from build123d import *

# Parameters (mm, degrees)
F0_W      = 24.5
F0_H      = 24.5
F1_DEPTH  = 58
F2_W      = 20.3
F2_H      = 20.3
F3_DEPTH  = 6
F4_W      = 20.5
F4_H      = 20.5
F5_DEPTH  = 30
F7_D      = 5.5
F8_W      = 6.4
F8_H      = 10
F9_DEPTH  = 25
F10_DEPTH = 5
F11_DEPTH = 0.25
F12_DEPTH = 0.25
F13_DEPTH = 1.5
F14_DEPTH = 1
F15_DEPTH = 1
F16_DEPTH = 2


with BuildPart() as f1:
    # F0 (on Top) → F1 (new body)
    with BuildSketch(Plane.XY):
        Rectangle(F0_W, F0_H)
    extrude(amount=F1_DEPTH)

    # F2 (on face) → F3 (cut)
    with BuildSketch(Plane(origin=(0, 0, 0), x_dir=(1, 0, 0), z_dir=(0, 0, -1))):
        Rectangle(F2_W, F2_H)
    extrude(amount=-F3_DEPTH, mode=Mode.SUBTRACT)

    # F4 (on face) → F5 (cut)
    with BuildSketch(Plane.XY.offset(58)):
        with Locations((2, 2)):
            Rectangle(F4_W, F4_H)
    extrude(amount=-F5_DEPTH, mode=Mode.SUBTRACT)

    # F7 (through all)
    with Locations(Plane.YZ.offset(-8.25)):
        with Locations((2, 43)):
            Hole(F7_D / 2)

    # F8 (on face) → F9 (cut)
    with BuildSketch(Plane(origin=(0, -8.25, 0), x_dir=(-1, 0, 0), z_dir=(0, 1, 0))):
        with Locations((-2.0447701301, 43.8107866645)):
            Rectangle(F8_W, F8_H)
    extrude(amount=-F9_DEPTH, mode=Mode.SUBTRACT)

    # F10 (add): a face of the model
    f10_faces = [f1.faces().sort_by_distance(p)[0] for p in [
        (2, 2, 28),
    ]]
    extrude(f10_faces, amount=F10_DEPTH)

    # F11 (cut): a face of the model
    f11_faces = [f1.faces().sort_by_distance(p)[0] for p in [
        (-1.1552298699, -10.25, 43.8107866645),
    ]]
    extrude(f11_faces, amount=-F11_DEPTH, mode=Mode.SUBTRACT)

    # F12 (cut): a face of the model
    f12_faces = [f1.faces().sort_by_distance(p)[0] for p in [
        (5.2447701301, -10.25, 43.8107866645),
    ]]
    extrude(f12_faces, amount=-F12_DEPTH, mode=Mode.SUBTRACT)

    # F13 (cut): a face of the model
    f13_faces = [f1.faces().sort_by_distance(p)[0] for p in [
        (2.0447701301, -10.25, 48.8107866645),
    ]]
    extrude(f13_faces, amount=-F13_DEPTH, mode=Mode.SUBTRACT)

    # F14 (cut): a face of the model
    f14_faces = [f1.faces().sort_by_distance(p)[0] for p in [
        (-12.25, -0.0340074224, 28.7619480432),
    ]]
    extrude(f14_faces, amount=-F14_DEPTH, mode=Mode.SUBTRACT)

    # F15 (cut): a face of the model
    f15_faces = [f1.faces().sort_by_distance(p)[0] for p in [
        (0.4045086201, -12.25, 28.0380957256),
    ]]
    extrude(f15_faces, amount=-F15_DEPTH, mode=Mode.SUBTRACT)

    # F16 (cut): a face of the model
    f16_faces = [f1.faces().sort_by_distance(p)[0] for p in [
        (0, 0, 6),
    ]]
    extrude(f16_faces, amount=-F16_DEPTH, mode=Mode.SUBTRACT)


solid = f1.part
Model file for the job. Use its own axes, mm. A direction names the side the tool comes from. Give positions to 0.01 mm unless a question says otherwise; leave off trailing zeros. Order: outer loops, then holes, each group sorted by start corner. A loop starts at its lowest first (then second) coordinate and runs counter-clockwise, first axis right, second up. Notation, with made-up numbers: (83.5, -29) - (106.5, -29) arc R29 cw to (106.5, -1) - close; hole circle Ø5 at (57.25, 17). An arc over 180 degrees is marked (long way). Write item = value, one per line. Start each with the question number.
1. Cut at B-B, the plane y = 2. List the corners of the cut face in (x, z), and give its area (3 significant figures).
2. Probe line 1 along Z through (x, y) = (-10.2, 2); line 2 along Z through (x, y) = (-9.5, 2); line 3 along Y through (x, z) = (8.5, 4.5). List the from-to ranges inside material, lowest first.
3. Drop flat-ended pins along their axis: P1, Ø10, axis at x = 3.5, y = 2, coming from the -Z side; P2, Ø1, axis at x = -5.5, y = -5, coming from the +Z side; P3, Ø5, axis at x = 9, y = -3.5, coming from the -Z side. Give the stop position or say it passes through.
4. Two-plate mould, pull along X, no slides. Class faces 1 (the flat face through (11, 2, 0)), 2 (the flat face through (10.15, 0, 4)), 3 (the flat face through (-8.25, 0, 46)): pulls with the +X half, pulls with the -X half, needs draft (parallel to the pull), parting line crosses it, or undercut.
5. Cut at C-C, the plane x = 1.25. List the corners of the cut face in (y, z), and give its area (3 significant figures).
6. Which spindle directions (+Z, -Z, +X, -X, +Y, -Y) get a long thin tool onto all of the face, cutting with end or side? Do faces 4 (the flat face through (2, -10, 50.311)), 5 (the flat face through (0, -10.15, 4)), 6 (the flat face through (-3, -8.25, 46)), 7 (the flat face through (0, 12.25, 16)). Say none if no direction does.
7. Cut at D-D, the plane z = 6. List the corners of the cut face in (x, y).
8. Cut at A-A, the plane z = 43. List the corners of the cut face in (x, y), and give its area (3 significant figures).
Taken from the geometry:
q1.outline = (-11.25, 0) - (-10.15, 0) - (-10.15, 8) - (10.15, 8) - (10.15, 0) - (12.25, 0) - (12.25, 33) - (-8.25, 33) - (-8.25, 40.25) - (-11.25, 40.25) - close; (-11.25, 45.75) - (-8.25, 45.75) - (-8.25, 58) - (-11.25, 58) - close
q1.area = 672 mm²
q2.line_1 = 0 to 40.25, 45.75 to 58
q2.line_2 = 8 to 40.25, 45.75 to 58
q2.line_3 = -11.25 to -10.15, 10.15 to 12.25
q3.P1 = 8
q3.P2 = 33
q3.P3 = 0
q4.face_1 = needs draft
q4.face_2 = undercut
q4.face_3 = pulls with the +X half
q5.outline = (-11.25, 0) - (-10.15, 0) - (-10.15, 8) - (10.15, 8) - (10.15, 0) - (12.25, 0) - (12.25, 33) - (-8.25, 33) - (-8.25, 38.81) - (-11.25, 38.81) - close; (-11.25, 50.31) - (-8.25, 50.31) - (-8.25, 58) - (-11.25, 58) - close
q5.area = 654 mm²
q6.face_4 = +Y, -Y
q6.face_5 = -Z
q6.face_6 = +Z, +X, +Y
q6.face_7 = +Z, -Z, +X, -X, +Y
q7.outline = (-11.25, -11.25) - (12.25, -11.25) - (12.25, 12.25) - (-11.25, 12.25) - close; hole (-10.15, -10.15) - (10.15, -10.15) - (10.15, 10.15) - (-10.15, 10.15) - close
q8.outline = (-11.25, -11.25) - (-1.41, -11.25) - (-1.41, -8.25) - (-8.25, -8.25) - (-8.25, -0.75) - (-11.25, -0.75) - close; (-11.25, 4.75) - (-8.25, 4.75) - (-8.25, 12.25) - (-11.25, 12.25) - close; (5.49, -11.25) - (12.25, -11.25) - (12.25, -8.25) - (5.49, -8.25) - close
q8.area = 94.8 mm²
